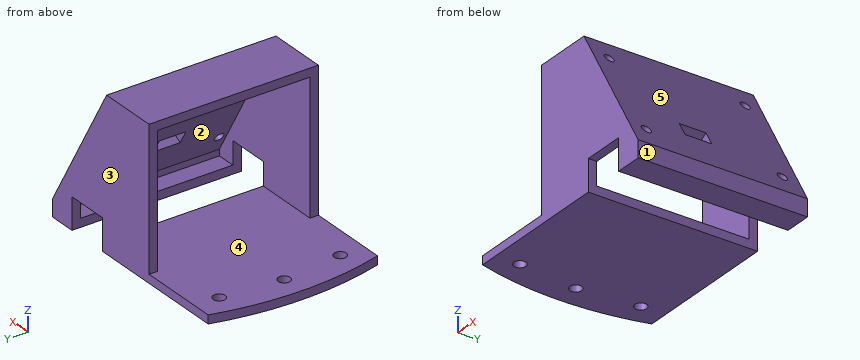
```python
from build123d import *

# Parameters (mm, degrees)
BOSS_EXTRUDE5_DEPTH            = 31.75
BOSS_EXTRUDE5_DEPTH_BACK       = 31.75
SKETCH1_R                      = 2.2479
BOSS_EXTRUDE6_DEPTH            = 3.175
SHELL2_START                   = -28.575
SHELL2_DEPTH                   = 57.15
F_1_0MM_DOWEL_HOLE1_AT_2_COUNT = 2
F_1_0MM_DOWEL_HOLE1_AT_2_PITCH = 51
F_1_0MM_DOWEL_HOLE1_AT_3_COUNT = 2
F_1_0MM_DOWEL_HOLE1_AT_3_PITCH = 64.202803677
F_1_0MM_DOWEL_HOLE1_AT_4_COUNT = 2
F_1_0MM_DOWEL_HOLE1_AT_4_PITCH = 39
SKETCH9_W                      = 16
SKETCH9_H                      = 9.25
SKETCH9_H_2                    = 2.52847891
CUT_EXTRUDE1_DEPTH             = 146.121062048
SKETCH10_W                     = 6
SKETCH10_H                     = 10
CUT_EXTRUDE2_DEPTH             = 3.175


# Read off the part's stored shape, not the designer's step: Shell2
with BuildPart() as part:
    # Sketch5 → Boss-Extrude5 (new, two sides: drawn at the far end of the back side and taken through both)
    with BuildSketch(Plane(origin=(0, 0, 0), x_dir=(1, 0, 0), z_dir=(0, 1, 0)).offset(-BOSS_EXTRUDE5_DEPTH_BACK)):
        Polygon((-31.75, 0), (-31.75, -6.35), (-60.25, -55.713448016), (-82.55, -55.713448016), (-82.55, 0), align=None)
    extrude(amount=BOSS_EXTRUDE5_DEPTH + BOSS_EXTRUDE5_DEPTH_BACK)

    # Sketch1 → Boss-Extrude6 (add)
    with BuildSketch(Plane.XY):
        with BuildLine():
            Line((-31.75, 31.75), (-113.647797428, 31.75))
            ThreePointArc((-113.647797428, 31.75), (-117.99951, 0), (-113.647797428, -31.75))
            Line((-113.647797428, -31.75), (-31.75, -31.75))
            Line((-31.75, -31.75), (-31.75, 31.75))
        make_face()
        with Locations((-106.71590324, -22.683165468)):
            Circle(SKETCH1_R, mode=Mode.SUBTRACT)
        with Locations((-109.1, 0)):
            Circle(SKETCH1_R, mode=Mode.SUBTRACT)
        with Locations((-106.71590324, 22.683165468)):
            Circle(SKETCH1_R, mode=Mode.SUBTRACT)
    extrude(amount=BOSS_EXTRUDE6_DEPTH)

    # Shell2 outline → Shell2 (cut)
    with BuildSketch(Plane(origin=(0, 0, 0), x_dir=(1, 0, 0), z_dir=(0, 1, 0)).offset(SHELL2_START)):
        Polygon((-34.925, -3.175), (-82.55, -3.175), (-82.55, -52.538448016), (-62.083087105, -52.538448016), (-34.925, -5.499261314), align=None)
    extrude(amount=SHELL2_DEPTH, mode=Mode.SUBTRACT)

    # Sketch8 → Ø1.0mm Dowel Hole1 (revolve, cut)
    with BuildSketch(Plane(origin=(-55.75, -25.5, 47.919219382), x_dir=(0.4999999999999977, 0, -0.86602540378444), z_dir=(0, 1, 0))):
        Polygon((0, 0), (0, 4.256549114), (1.8, 3.175), (1.8, 0), align=None)
    f_1_0mm_dowel_hole1 = revolve(axis=Axis((-50.250738686, -25.5, 51.094219382), (-0.86602540378444, 0, -0.4999999999999977)), mode=Mode.SUBTRACT)

    # Ø1.0mm Dowel Hole1 at 2: Ø1.0mm Dowel Hole1 ×2
    with Locations(*[(0, i * F_1_0MM_DOWEL_HOLE1_AT_2_PITCH, 0) for i in range(1, F_1_0MM_DOWEL_HOLE1_AT_2_COUNT)]):
        add(f_1_0mm_dowel_hole1, mode=Mode.SUBTRACT)

    # Ø1.0mm Dowel Hole1 at 3: Ø1.0mm Dowel Hole1 ×2
    with Locations(*[Vector(0.3037250537853972, 0.7943578329771961, -0.5260672246879011) * (i * F_1_0MM_DOWEL_HOLE1_AT_3_PITCH) for i in range(1, F_1_0MM_DOWEL_HOLE1_AT_3_COUNT)]):
        add(f_1_0mm_dowel_hole1, mode=Mode.SUBTRACT)

    # Ø1.0mm Dowel Hole1 at 4: Ø1.0mm Dowel Hole1 ×2
    with Locations(*[Vector(0.49999999999999767, 0, -0.86602540378444) * (i * F_1_0MM_DOWEL_HOLE1_AT_4_PITCH) for i in range(1, F_1_0MM_DOWEL_HOLE1_AT_4_COUNT)]):
        add(f_1_0mm_dowel_hole1, mode=Mode.SUBTRACT)

    # Sketch9 → Cut-Extrude1 (cut, through all)
    with BuildSketch(Plane.XZ.offset(31.75)):
        with Locations((-50, 4.625)):
            Rectangle(SKETCH9_W, SKETCH9_H)
        with Locations((-50, 10.514239455)):
            Rectangle(SKETCH9_W, SKETCH9_H_2)
    extrude(amount=-CUT_EXTRUDE1_DEPTH, mode=Mode.SUBTRACT)

    # Sketch10 → Cut-Extrude2 (cut)
    with BuildSketch(Plane(origin=(-21.062869343, 0, -12.160653285), x_dir=(-0.4999999999999977, 0, 0.8660254037844399), z_dir=(-0.8660254037844399, 0, -0.4999999999999977))):
        with Locations((38.874261314, -4)):
            Rectangle(SKETCH10_W, SKETCH10_H)
    extrude(amount=CUT_EXTRUDE2_DEPTH, mode=Mode.SUBTRACT)


solid = part.part
```
CAD build for the part. Positions are in the model's coordinates, mm. Face numbers are marked on the shaded views. A direction names the side the tool comes from. Give positions to 0.01 mm unless a question says otherwise; leave off trailing zeros. Order: outer loops, then holes, each group sorted by start corner. A loop starts at its lowest first (then second) coordinate and runs counter-clockwise, first axis right, second up. Notation, with made-up numbers: M -19.75,19.5 L 17.25,19.5 A31 cw 17.25,57.5 Z; hole C -2,81.25 d11. An arc over 180 degrees is marked long. Put each result on its own line as item: value. Start each with the question number.
(1) Saw through at D-D, the plane y = 11.5. Write the cut outline in (x, z) (3 decimals).
(2) Which spindle directions (+Z, -Z, +X, -X, +Y, -Y) get a long thin tool onto all of the face, cutting with end or side? Do the marked faces 1 and 2. Say none if no direction does.
(3) Drill centre lines: line 1 along Y through (x, z) = (-71.5, 42.5) (3 decimals); line 2 along Z through (x, y) = (-73, -3) (3 decimals); line 3 along Z through (x, y) = (-59, 28) (3 decimals). Where is each one in solid material? Low to high.
(4) Mould opens along Y. For the marked faces 3, 4 and 5 say: +Y half, -Y half, draft (parallel to the pull), parting line (faces both ways), or undercut.
(5) Saw through at C-C, the plane x = -66.5. Write the cut outline in (y, z) (3 decimals).
(6) Saw through at B-B, the plane z = 4.5. Write the cut outline in (x, y) (3 decimals).
(7) Saw through at A-A, the plane y = 0. Give the number of separate pieces and of enclosed holes in the cut face, then the cut area to 3 significant figures.
(8) Flat gauge pins, fed straight in: pin 1 Ø5 at (x, y) = (-96.5, 24.5) entering from +Z (3 decimals); pin 2 Ø4 at (y, z) = (-14.5, 9.5) entering from -X; pin 3 Ø10 at (y, z) = (-10.5, 35) entering from -X; pin 4 Ø3.5 at (x, y) = (-106.72, -22.68) entering from +Z. Where does each tip first touch, or does it go through?
Check result:
1. outline: M -117.438,0 L -58,0 L -58,3.175 L -117.438,3.175 Z; M -82.55,52.538 L -62.083,52.538 L -34.925,5.499 L -34.925,3.175 L -42,3.175 L -42,0 L -31.75,0 L -31.75,6.35 L -60.25,55.713 L -82.55,55.713 Z
2. face 1: +Z, -Z, +X, +Y, -Y
2. face 2: -X
3. line 1: y = -31.75 to -28.575, 28.575 to 31.75
3. line 2: z = 0 to 3.175, 52.538 to 55.713
3. line 3: z = 0 to 3.175, 47.198 to 53.548
4. face 3: +Y half
4. face 4: undercut
4. face 5: draft
5. outline: M -31.75,0 L 31.75,0 L 31.75,55.713 L -31.75,55.713 Z; hole M -28.575,3.175 L 28.575,3.175 L 28.575,52.538 L -28.575,52.538 Z
6. outline: M -82.55,-31.75 L -58,-31.75 L -58,-28.575 L -82.55,-28.575 Z; M -82.55,28.575 L -58,28.575 L -58,31.75 L -82.55,31.75 Z; M -42,-31.75 L -31.75,-31.75 L -31.75,31.75 L -42,31.75 L -42,28.575 L -34.925,28.575 L -34.925,-28.575 L -42,-28.575 Z
7. separate pieces: 4
7. enclosed holes: 0
7. area: 443 mm2
8. pin 1: stops at z = 3.175
8. pin 2: stops at x = -38.39
8. pin 3: stops at x = -54.84
8. pin 4: passes through
